The listing builds one solid part. Answer for the finished solid, in the listing's coordinates (mm). Face numbers are marked on the shaded views. A direction names the side the tool comes from. Give positions to 0.01 mm unless a question says otherwise; leave off trailing zeros. Write each loop counter-clockwise with the first axis right and the second up, starting at its lowest first coordinate (ties: lowest second). Pieces come first, ordered by that corner, then holes. Notation, with made-up numbers: (33, 56.25) - (83, 56.25) arc R19 cw to (83, 83.25) - close; hole circle Ø3 at (-28, -29.5). An arc over 180 degrees is marked (long way). Answer in a Markdown table with one row per item. Add a question column.
from build123d import *

# Parameters (mm, degrees)
F1_DEPTH       = 6.35
F3_DEPTH       = 6.35
F5_D           = 2.032
F5_CSINK_D     = 3.175
F5_CSINK_ANGLE = 82
F7_D           = 2.032


with BuildPart() as f1:
    # F0 (on Front) → F1 (new body)
    with BuildSketch(Plane.XZ):
        with BuildLine():
            ThreePointArc((-5.08, 12.7), (-3.5921024484, 9.1078975516), (0, 7.62))
            Line((0, 7.62), (0, 12.7))
            Line((0, 12.7), (0, 17.78))
            ThreePointArc((0, 17.78), (-3.5921024484, 16.2921024484), (-5.08, 12.7))
        make_face()
        with BuildLine():
            Line((0, 12.7), (0, 7.62))
            ThreePointArc((0, 7.62), (3.5921024484, 9.1078975516), (5.08, 12.7))
            ThreePointArc((5.08, 12.7), (3.5921024484, 16.2921024484), (0, 17.78))
            Line((0, 17.78), (0, 12.7))
        make_face()
        with BuildLine():
            ThreePointArc((5.08, 12.7), (3.5921024484, 9.1078975516), (0, 7.62))
            ThreePointArc((0, 7.62), (-3.5921024484, 9.1078975516), (-5.08, 12.7))
            Line((-5.08, 12.7), (-5.08, 0))
            ThreePointArc((-5.08, 0), (0, -5.08), (5.08, 0))
            Line((5.08, 0), (5.08, 12.7))
        make_face()
        with BuildLine():
            ThreePointArc((0, 17.78), (3.5921024484, 16.2921024484), (5.08, 12.7))
            Line((5.08, 12.7), (5.08, 32.7368881382))
            Line((5.08, 32.7368881382), (4.2115108686, 31.4493000504))
            ThreePointArc((4.2115108686, 31.4493000504), (2.384915539, 29.8046262283), (0, 29.21))
            Line((0, 29.21), (0, 17.78))
        make_face()
        with BuildLine():
            Line((-5.08, 34.29), (-5.08, 12.7))
            ThreePointArc((-5.08, 12.7), (-3.5921024484, 16.2921024484), (0, 17.78))
            Line((0, 17.78), (0, 29.21))
            ThreePointArc((0, 29.21), (-3.5921024484, 30.6978975516), (-5.08, 34.29))
        make_face()
        with BuildLine():
            Line((4.2115108686, 31.4493000504), (5.08, 32.7368881382))
            Line((5.08, 32.7368881382), (5.08, 34.29))
            ThreePointArc((5.08, 34.29), (4.4853737717, 36.674915539), (2.8406999496, 38.5015108686))
            Line((2.8406999496, 38.5015108686), (0, 34.29))
            Line((0, 34.29), (0, 29.21))
            ThreePointArc((0, 29.21), (2.384915539, 29.8046262283), (4.2115108686, 31.4493000504))
        make_face()
        with BuildLine():
            Line((5.08, 34.29), (5.08, 32.7368881382))
            Line((5.08, 32.7368881382), (26.9371104656, 65.141386999))
            ThreePointArc((26.9371104656, 65.141386999), (25.5662995467, 72.1935978172), (18.5140887285, 70.8227868983))
            Line((18.5140887285, 70.8227868983), (-4.2115108686, 37.1306999496))
            ThreePointArc((-4.2115108686, 37.1306999496), (-0.9693096965, 39.2766660919), (2.8406999496, 38.5015108686))
            ThreePointArc((2.8406999496, 38.5015108686), (4.4853737717, 36.674915539), (5.08, 34.29))
        make_face()
        with BuildLine():
            ThreePointArc((-4.2115108686, 37.1306999496), (-4.8580281603, 35.77524826), (-5.08, 34.29))
            ThreePointArc((-5.08, 34.29), (-3.5921024484, 30.6978975516), (0, 29.21))
            Line((0, 29.21), (0, 34.29))
            Line((0, 34.29), (2.8406999496, 38.5015108686))
            ThreePointArc((2.8406999496, 38.5015108686), (-0.9693096965, 39.2766660919), (-4.2115108686, 37.1306999496))
        make_face()
    extrude(amount=F1_DEPTH)

    # F2 (on face) → F3 (join)
    with BuildSketch(Plane.XZ.offset(6.35)):
        with BuildLine():
            ThreePointArc((0, 8.89), (2.6940768363, 10.0059231637), (3.81, 12.7))
            ThreePointArc((3.81, 12.7), (-2.6940768363, 15.3940768363), (0, 8.89))
        make_face()
    extrude(amount=F3_DEPTH)

    # F5 (through all)
    with Locations(Plane.XZ.offset(12.7)):
        with Locations((0, 12.7)):
            CounterSinkHole(F5_D / 2, F5_CSINK_D / 2, counter_sink_angle=F5_CSINK_ANGLE)

    # F7 (through all)
    with Locations(Plane.XZ.offset(6.35)):
        with Locations((0, 0)):
            Hole(F7_D / 2)


solid = f1.part
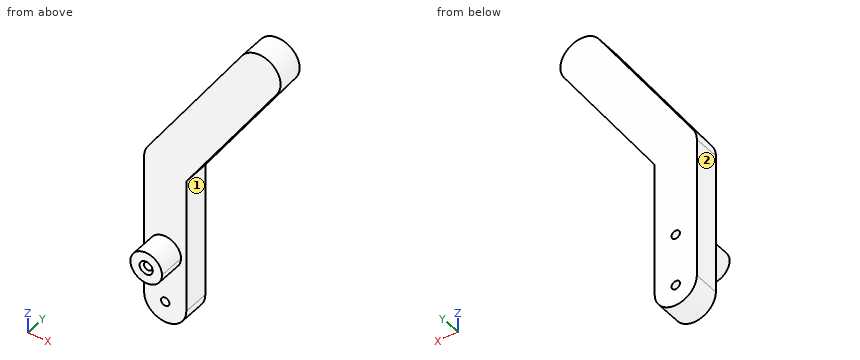
1. Section D-D (x = 16) is taken. Give the vertices of the cut face in (y, z).
2. Section A-A (x = -2.5) is taken. Give the vertices of the cut face in (y, z), and give its area (3 significant figures).
3. A tool of negligible diameter and unlimited length cuts with its end or side. For the marked faces 1 and 2, from which of +Z, -Z, +X, -X, +Y, -Y can it reach the whole face along a straight path? Write none if from no direction.
4. Section C-C (x = 2.5) is taken. Give the vertices of the cut face in (y, z), and give its area (3 significant figures).
5. Given pin 1 Ø3 at (x, y) = (10, -4) entering from -Z; pin 2 Ø2.5 at (x, z) = (0, 12.7) entering from +Y; pin 3 Ø1 at (y, z) = (-1.5, 57) entering from +X; pin 4 Ø2 at (x, y) = (11, -8.5) entering from +Z, each flat-ended and moving along its own axis, determine where each tip first touches the part or whether it passes through.
6. Straight lines are drawn through the part: L1, parallel to Z at x = 0, y = -3.75; L2, parallel to X at y = -7.75, z = 12.7; L3, parallel to Y at x = 11.5, z = 52. For each, find the intervals that lie inside material, in ascending order. Write a range as [from, to].
7. Section B-B (z = 35) is taken. Give the vertices of the cut face in (x, y).
Geometry check:
| question | item | result |
|---|---|---|
| 1 | outline | (-6.35, 48.93) - (0, 48.93) - (0, 67.1) - (-6.35, 67.1) - close |
| 2 | outline | (-12.7, 9.82) - (-6.35, 9.82) - (-6.35, -4.42) - (0, -4.42) - (0, 39.67) - (-6.35, 39.67) - (-6.35, 15.58) - (-12.7, 15.58) - close |
| 2 | area | 316 mm² |
| 3 | face 1 | -Z, +X, +Y, -Y |
| 3 | face 2 | +Z, -Z, -X, +Y, -Y |
| 4 | outline | (-12.7, 9.82) - (-6.35, 9.82) - (-6.35, -4.42) - (0, -4.42) - (0, 47.08) - (-6.35, 47.08) - (-6.35, 15.58) - (-12.7, 15.58) - close |
| 4 | area | 364 mm² |
| 5 | pin 1 | z = 37.81 |
| 5 | pin 2 | y = 0 |
| 5 | pin 3 | x = 21.78 |
| 5 | pin 4 | through |
| 6 | L1 | [-5.08, -1.02], [1.02, 11.68], [13.72, 43.37] |
| 6 | L2 | [-3.81, -1.02], [1.02, 3.81] |
| 6 | L3 | [-6.35, 0] |
| 7 | outline | (-5.03, -6.35) - (6.61, -6.35) - (6.61, 0) - (-5.03, 0) - close |
